Check sheet for the modelled part. Datum: model origin and axes. Units: mm. A direction names the side the tool comes from. Round coordinates to 2 decimals unless told otherwise and drop trailing zeros. Loops run counter-clockwise (first coordinate to the right, second up) from the corner with the lowest first, then second, coordinate; pieces in that order, holes last. Notation, with made-up numbers: (-19, -2) - (-7, -2) arc R20 ccw to (-7, 14) - close; hole circle Ø5 at (72, 1.25). An arc over 180 degrees is marked (long way). Return JSON: item names as keys, results as strings.
from build123d import *

# Parameters (mm, degrees)
SKETCH1_R                      = 14.6812
SKETCH1_R_2                    = 11.5062
BEARING_INSERT_EXTRUDE_DEPTH   = 4.7625
APEX_SLOT_INSERT_EXTRUDE_DEPTH = 3.175
FILLET1_R                      = 5.08
FILLET2_R                      = 2.54
FILLET3_R                      = 3.81


with BuildPart() as part:
    # Sketch1 → Bearing_Insert_Extrude (new, symmetric)
    with BuildSketch(Plane(origin=(0, 0, 0), x_dir=(1, 0, 0), z_dir=(0, 1, 0))):
        with Locations(Location((0, 0, 0), (0, 0, 90))):
            Circle(SKETCH1_R)
        with Locations(Location((0, 0, 0), (0, 0, 90))):
            Circle(SKETCH1_R_2, mode=Mode.SUBTRACT)
    extrude(amount=BEARING_INSERT_EXTRUDE_DEPTH, both=True)

    # Sketch1<4> → Apex_Slot_Insert_Extrude (add, symmetric)
    # profile 1 of 2: a face of its own
    with BuildSketch(Plane(origin=(0, 0, 0), x_dir=(1, 0, 0), z_dir=(0, 1, 0))):
        with BuildLine():
            Line((-10.31875, -10.443228997), (-10.31875, -66.04))
            Line((-10.31875, -66.04), (10.31875, -66.04))
            Line((10.31875, -66.04), (10.31875, -37.376828003))
            Line((10.31875, -37.376828003), (25.024230745, -61.980207141))
            Line((25.024230745, -61.980207141), (42.738677597, -51.392252712))
            Line((42.738677597, -51.392252712), (14.215063896, -3.670094259))
            ThreePointArc((14.215063896, -3.670094259), (3.906936657, -14.151801278), (-10.31875, -10.443228997))
        make_face()
        with BuildLine():
            ThreePointArc((5.55625, -55.72125), (0, -61.2775), (-5.55625, -55.72125))
            Line((-5.55625, -55.72125), (-5.55625, -35.40125))
            ThreePointArc((-5.55625, -35.40125), (0, -29.845), (5.55625, -35.40125))
            Line((5.55625, -35.40125), (5.55625, -55.72125))
        make_face(mode=Mode.SUBTRACT)
        with BuildLine():
            ThreePointArc((33.356751109, -44.978403385), (31.438080072, -52.598280653), (23.818202804, -50.679609616))
            Line((23.818202804, -50.679609616), (13.393139982, -33.237692715))
            ThreePointArc((13.393139982, -33.237692715), (15.31181102, -25.617815447), (22.931688287, -27.536486485))
            Line((22.931688287, -27.536486485), (33.356751109, -44.978403385))
        make_face(mode=Mode.SUBTRACT)
    # profile 2 of 2: a face of its own
    with BuildSketch(Plane(origin=(0, 0, 0), x_dir=(1, 0, 0), z_dir=(0, 1, 0))):
        with BuildLine():
            Line((-10.31875, -10.443228997), (-10.31875, -66.04))
            Line((-10.31875, -66.04), (10.31875, -66.04))
            Line((10.31875, -66.04), (10.31875, -37.376828003))
            Line((10.31875, -37.376828003), (25.024230745, -61.980207141))
            Line((25.024230745, -61.980207141), (42.738677597, -51.392252712))
            Line((42.738677597, -51.392252712), (14.215063896, -3.670094259))
            ThreePointArc((14.215063896, -3.670094259), (3.906936657, -14.151801278), (-10.31875, -10.443228997))
        make_face()
        with BuildLine():
            ThreePointArc((5.55625, -55.72125), (0, -61.2775), (-5.55625, -55.72125))
            Line((-5.55625, -55.72125), (-5.55625, -35.40125))
            ThreePointArc((-5.55625, -35.40125), (0, -29.845), (5.55625, -35.40125))
            Line((5.55625, -35.40125), (5.55625, -55.72125))
        make_face(mode=Mode.SUBTRACT)
        with BuildLine():
            ThreePointArc((33.356751109, -44.978403385), (31.438080072, -52.598280653), (23.818202804, -50.679609616))
            Line((23.818202804, -50.679609616), (13.393139982, -33.237692715))
            ThreePointArc((13.393139982, -33.237692715), (15.31181102, -25.617815447), (22.931688287, -27.536486485))
            Line((22.931688287, -27.536486485), (33.356751109, -44.978403385))
        make_face(mode=Mode.SUBTRACT)
    extrude(amount=APEX_SLOT_INSERT_EXTRUDE_DEPTH, both=True)

    # Fillet1
    fillet1_edges = [part.edges().sort_by_distance(p)[0] for p in [
        (14.215063896, 0, 3.670094259),
        (-10.31875, 0, 10.443228997),
    ]]
    fillet(fillet1_edges, radius=FILLET1_R)

    # Fillet2
    fillet2_edges = [part.edges().sort_by_distance(p)[0] for p in [
        (-10.31875, 0, 66.04),
        (10.31875, 0, 66.04),
        (25.024230745, 0, 61.980207141),
        (42.738677597, 0, 51.392252712),
    ]]
    fillet(fillet2_edges, radius=FILLET2_R)

    # Fillet3
    fillet3_edges = [part.edges().sort_by_distance(p)[0] for p in [
        (10.31875, 0, 37.376828003),
    ]]
    fillet(fillet3_edges, radius=FILLET3_R)


solid = part.part
Q1. Draft check along X on faces 1 (the face through (-10.615, -0.044, 10.674)), 2 (the face through (9.55, 0.04, 65.32)), 3 (the face through (31.542, 0.044, 52.534)). Enter one of: released by +X, released by -X, zero draft, split by the parting line, or undercut.
Answer key:
{"face 1": "released by -X", "face 2": "released by +X", "face 3": "undercut"}
Q2. Tool access check on faces 4 (the face through (-10.319, 0, 38)), 5 (the face through (14.59, -0.04, 3.72)), 6 (the face through (0.122, 0.044, 61.276)), 7 (the face through (20.516, 0.044, 54.437)). Record the directions out of +Z, -Z, +X, -X, +Y, -Y that give a thin tool (end or side, any length) a straight path to the whole face; none if there is none.
Answer key:
{"face 4": "+Z, -X, +Y, -Y", "face 5": "+X, +Y, -Y", "face 6": "+Y, -Y", "face 7": "+Z, +Y, -Y"}
Q3. Sectioned sample at B-B (x = 0). Enter the section's corners in (y, z) (1 decimal).
Answer key:
{"outline": "(-4.8, -14.7) - (4.8, -14.7) - (4.8, -11.5) - (-4.8, -11.5) - close; (-4.8, 11.5) - (4.8, 11.5) - (4.8, 14.7) - (3.2, 14.7) - (3.2, 29.8) - (-3.2, 29.8) - (-3.2, 14.7) - (-4.8, 14.7) - close; (-3.2, 61.3) - (3.2, 61.3) - (3.2, 66) - (-3.2, 66) - close"}
Q4. Sectioned sample at D-D (z = 43). Enter the section's corners in (x, y) (3 decimals), plus the area to 3 significant figures.
Answer key:
{"outline": "(-10.319, -3.175) - (-5.556, -3.175) - (-5.556, 3.175) - (-10.319, 3.175) - close; (5.556, -3.175) - (19.228, -3.175) - (19.228, 3.175) - (5.556, 3.175) - close; (32.174, -3.175) - (37.723, -3.175) - (37.723, 3.175) - (32.174, 3.175) - close", "area": "152 mm²"}
Q5. Scan lines: probe 1 along X at (y, z) = (-2.5, 0); probe 2 along X at (y, z) = (-1.25, 42); probe 3 along Z at (x, y) = (3.5, -1.5). Record each from-to range of solid material in increasing order. Write a range as [from, to].
Answer key:
{"probe 1": "x = [-14.68, -11.51], [11.51, 14.68]", "probe 2": "x = [-10.32, -5.56], [5.56, 18.63], [31.58, 37.12]", "probe 3": "z = [-14.26, -10.96], [10.96, 31.09], [60.04, 66.04]"}
Q6. Depth check by flat-ended pin: P1, Ø3, axis at x = 25.5, z = 26.5, coming from the -Y side (3 decimals); P2, Ø1.5, axis at y = -0.5, z = 11.5, coming from the -X side; P3, Ø12, axis at x = 23.5, z = 46.5, coming from the +Y side (3 decimals). Enter the tip coordinate at first touch or a pass-through.
Answer key:
{"P1": "stops at y = -3.175", "P2": "stops at x = -10.59", "P3": "stops at y = 3.175"}
Q7. Sectioned sample at C-C (x = 22). Enter the section's corners in (y, z) (3 decimals).
Answer key:
{"outline": "(-3.175, 16.695) - (3.175, 16.695) - (3.175, 26.369) - (-3.175, 26.369) - close; (-3.175, 47.638) - (3.175, 47.638) - (3.175, 56.92) - (-3.175, 56.92) - close"}
Q8. Sectioned sample at A-A (z = 0). Enter the section's corners in (x, y), plus the area to 3 significant figures.
Answer key:
{"outline": "(-14.68, -4.76) - (-11.51, -4.76) - (-11.51, 4.76) - (-14.68, 4.76) - close; (11.51, -4.76) - (14.68, -4.76) - (14.68, 4.76) - (11.51, 4.76) - close", "area": "60.5 mm²"}
